The model under review builds one solid part; all positions refer to its coordinate system, in mm. Face numbers are marked on the shaded views. A direction names the side the tool comes from. Coordinates: 2 decimals unless noted, no trailing zeros. Order: outer loops, then holes, each group sorted by start corner. A loop starts at its lowest first (then second) coordinate and runs counter-clockwise, first axis right, second up. Notation, with made-up numbers: (-35.75, 38.5) - (5.25, 38.5) arc R33 cw to (5.25, 71.5) - close; hole circle Ø5 at (-33.5, 80). An arc over 180 degrees is marked (long way). Answer in a Markdown table with one row per item.
```python
from build123d import *

# Parameters (mm, degrees)
SKETCH1_W                = 47.8
SKETCH1_H                = 47.8
SKETCH1_W_2              = 40.2
SKETCH1_H_2              = 40.2
BOSS_EXTRUDE1_DEPTH      = 11
SKETCH3_W                = 20
SKETCH3_H                = 6
CUT_EXTRUDE1_DEPTH       = 55.562349656
SKETCH4_W                = 5
SKETCH4_H                = 6
CUT_EXTRUDE2_DEPTH       = 1
CUT_EXTRUDE4_REACH       = 56.562
SKETCH6_R                = 1.35
CUT_EXTRUDE5_REACH       = 56.562
SKETCH7_R                = 1.35
CUT_EXTRUDE6_REACH       = 56.562
SKETCH8_R                = 1.35
CUT_EXTRUDE7_REACH       = 56.562
SKETCH9_R                = 1.65
BOSS_EXTRUDE7_DEPTH      = 8
BOSS_EXTRUDE7_DEPTH_BACK = 10
SKETCH5_W                = 5
SKETCH5_H                = 6
CUT_EXTRUDE3_DEPTH       = 1.2
SKETCH11_R               = 2.6
CUT_EXTRUDE8_DEPTH       = 2


with BuildPart() as part:
    # Sketch1 → Boss-Extrude1 (new body)
    with BuildSketch(Plane(origin=(0, 0, 0), x_dir=(1, 0, 0), z_dir=(0, 1, 0))):
        Rectangle(SKETCH1_W, SKETCH1_H)
        Rectangle(SKETCH1_W_2, SKETCH1_H_2, mode=Mode.SUBTRACT)
    extrude(amount=BOSS_EXTRUDE1_DEPTH)

    # Sketch3 → Cut-Extrude1 (cut, through all)
    with BuildSketch(Plane.XY.offset(23.9)):
        with Locations((0, 3)):
            Rectangle(SKETCH3_W, SKETCH3_H)
    extrude(amount=-CUT_EXTRUDE1_DEPTH, mode=Mode.SUBTRACT)

    # Sketch4 → Cut-Extrude2 (cut)
    with BuildSketch(Plane.XY.offset(-20.1)):
        with Locations((-12.5, 3)):
            Rectangle(SKETCH4_W, SKETCH4_H)
        with Locations((12.5, 3)):
            Rectangle(SKETCH4_W, SKETCH4_H)
    extrude(amount=-CUT_EXTRUDE2_DEPTH, mode=Mode.SUBTRACT)

    # Sketch6 → Cut-Extrude4 (cut, up to next)
    with BuildSketch(Plane(origin=(0, 0, -23.9), x_dir=(-1, 0, 0), z_dir=(0, 0, -1)), mode=Mode.PRIVATE) as cut_extrude4_sk1:
        with Locations((-8.9, 9)):
            Circle(SKETCH6_R)
    cut_extrude4_tool1 = extrude(cut_extrude4_sk1.sketch, amount=-CUT_EXTRUDE4_REACH, mode=Mode.PRIVATE) & part.part
    # Sketch6 → Cut-Extrude4 (cut, up to next)
    with BuildSketch(Plane(origin=(0, 0, -23.9), x_dir=(-1, 0, 0), z_dir=(0, 0, -1)), mode=Mode.PRIVATE) as cut_extrude4_sk2:
        with Locations((8.9, 9)):
            Circle(SKETCH6_R)
    cut_extrude4_tool2 = extrude(cut_extrude4_sk2.sketch, amount=-CUT_EXTRUDE4_REACH, mode=Mode.PRIVATE) & part.part
    add(cut_extrude4_tool1.solids().sort_by_distance((8.9, 9, -23.9))[0], mode=Mode.SUBTRACT)
    add(cut_extrude4_tool2.solids().sort_by_distance((-8.9, 9, -23.9))[0], mode=Mode.SUBTRACT)

    # Sketch7 → Cut-Extrude5 (cut, up to next)
    with BuildSketch(Plane.XY.offset(23.9), mode=Mode.PRIVATE) as cut_extrude5_sk1:
        with Locations((9.4, 8.412816521)):
            Circle(SKETCH7_R)
    cut_extrude5_tool1 = extrude(cut_extrude5_sk1.sketch, amount=-CUT_EXTRUDE5_REACH, mode=Mode.PRIVATE) & part.part
    # Sketch7 → Cut-Extrude5 (cut, up to next)
    with BuildSketch(Plane.XY.offset(23.9), mode=Mode.PRIVATE) as cut_extrude5_sk2:
        with Locations((-5.6, 8.412816521)):
            Circle(SKETCH7_R)
    cut_extrude5_tool2 = extrude(cut_extrude5_sk2.sketch, amount=-CUT_EXTRUDE5_REACH, mode=Mode.PRIVATE) & part.part
    add(cut_extrude5_tool1.solids().sort_by_distance((9.4, 8.412817, 23.9))[0], mode=Mode.SUBTRACT)
    add(cut_extrude5_tool2.solids().sort_by_distance((-5.6, 8.412817, 23.9))[0], mode=Mode.SUBTRACT)

    # Sketch8 → Cut-Extrude6 (cut, up to next)
    with BuildSketch(Plane(origin=(23.9, 0, 0), x_dir=(0, 0, -1), z_dir=(1, 0, 0)), mode=Mode.PRIVATE) as cut_extrude6_sk1:
        with Locations((-11.9, 4)):
            Circle(SKETCH8_R)
    cut_extrude6_tool1 = extrude(cut_extrude6_sk1.sketch, amount=-CUT_EXTRUDE6_REACH, mode=Mode.PRIVATE) & part.part
    # Sketch8 → Cut-Extrude6 (cut, up to next)
    with BuildSketch(Plane(origin=(23.9, 0, 0), x_dir=(0, 0, -1), z_dir=(1, 0, 0)), mode=Mode.PRIVATE) as cut_extrude6_sk2:
        with Locations((-6.4, 4)):
            Circle(SKETCH8_R)
    cut_extrude6_tool2 = extrude(cut_extrude6_sk2.sketch, amount=-CUT_EXTRUDE6_REACH, mode=Mode.PRIVATE) & part.part
    # Sketch8 → Cut-Extrude6 (cut, up to next)
    with BuildSketch(Plane(origin=(23.9, 0, 0), x_dir=(0, 0, -1), z_dir=(1, 0, 0)), mode=Mode.PRIVATE) as cut_extrude6_sk3:
        with Locations(Location((6.4, 4, 0), (0, 0, 180))):
            Circle(SKETCH8_R)
    cut_extrude6_tool3 = extrude(cut_extrude6_sk3.sketch, amount=-CUT_EXTRUDE6_REACH, mode=Mode.PRIVATE) & part.part
    # Sketch8 → Cut-Extrude6 (cut, up to next)
    with BuildSketch(Plane(origin=(23.9, 0, 0), x_dir=(0, 0, -1), z_dir=(1, 0, 0)), mode=Mode.PRIVATE) as cut_extrude6_sk4:
        with Locations(Location((11.9, 4, 0), (0, 0, 180))):
            Circle(SKETCH8_R)
    cut_extrude6_tool4 = extrude(cut_extrude6_sk4.sketch, amount=-CUT_EXTRUDE6_REACH, mode=Mode.PRIVATE) & part.part
    add(cut_extrude6_tool1.solids().sort_by_distance((23.9, 4, 11.9))[0], mode=Mode.SUBTRACT)
    add(cut_extrude6_tool2.solids().sort_by_distance((23.9, 4, 6.4))[0], mode=Mode.SUBTRACT)
    add(cut_extrude6_tool3.solids().sort_by_distance((23.9, 4, -6.4))[0], mode=Mode.SUBTRACT)
    add(cut_extrude6_tool4.solids().sort_by_distance((23.9, 4, -11.9))[0], mode=Mode.SUBTRACT)

    # Sketch9 → Cut-Extrude7 (cut, up to next)
    with BuildSketch(Plane.ZY.offset(23.9), mode=Mode.PRIVATE) as cut_extrude7_sk1:
        with Locations((0, 6)):
            Circle(SKETCH9_R)
    cut_extrude7_tool1 = extrude(cut_extrude7_sk1.sketch, amount=-CUT_EXTRUDE7_REACH, mode=Mode.PRIVATE) & part.part
    add(cut_extrude7_tool1.solids().sort_by_distance((-23.9, 6, 0))[0], mode=Mode.SUBTRACT)

    # Sketch10 → Boss-Extrude7 (add, two sides: drawn at the far end of the back side and taken through both)
    with BuildSketch(Plane(origin=(23.9, 0, 0), x_dir=(0, 0, -1), z_dir=(1, 0, 0)).offset(-BOSS_EXTRUDE7_DEPTH_BACK)):
        with BuildLine():
            Line((-42.1, 0), (-20.1, 0))
            Line((-20.1, 0), (-20.1, 11))
            Line((-20.1, 11), (-25.535668372, 21.478172171))
            ThreePointArc((-25.535668372, 21.478172171), (-32.693052351, 5.7261976), (-46.3, 16.412816521))
            Line((-46.3, 16.412816521), (-46.3, 8.096211929))
            Line((-46.3, 8.096211929), (-42.1, 0))
        make_face()
        with BuildLine():
            ThreePointArc((-46.3, 16.412816521), (-32.693052351, 5.7261976), (-25.535668372, 21.478172171))
            Line((-25.535668372, 21.478172171), (-26.423334884, 21.017685293))
            ThreePointArc((-26.423334884, 21.017685293), (-32.930047592, 6.697708411), (-45.3, 16.412816521))
            Line((-45.3, 16.412816521), (-46.3, 16.412816521))
        make_face()
    extrude(amount=BOSS_EXTRUDE7_DEPTH + BOSS_EXTRUDE7_DEPTH_BACK)

    # Sketch5 → Cut-Extrude3 (cut)
    with BuildSketch(Plane(origin=(0, 0, 20.1), x_dir=(-1, 0, 0), z_dir=(0, 0, -1))):
        with Locations((-12.5, 3)):
            Rectangle(SKETCH5_W, SKETCH5_H)
        with Locations((12.5, 3)):
            Rectangle(SKETCH5_W, SKETCH5_H)
    extrude(amount=-CUT_EXTRUDE3_DEPTH, mode=Mode.SUBTRACT)

    # Sketch11 → Cut-Extrude8 (cut)
    with BuildSketch(Plane(origin=(23.9, 0, 0), x_dir=(0, 0, -1), z_dir=(1, 0, 0))):
        with Locations((11.9, 4)):
            Circle(SKETCH11_R)
        with Locations((6.4, 4)):
            Circle(SKETCH11_R)
        with Locations((-6.4, 4)):
            Circle(SKETCH11_R)
        with Locations((-11.9, 4)):
            Circle(SKETCH11_R)
    extrude(amount=-CUT_EXTRUDE8_DEPTH, mode=Mode.SUBTRACT)


solid = part.part
```
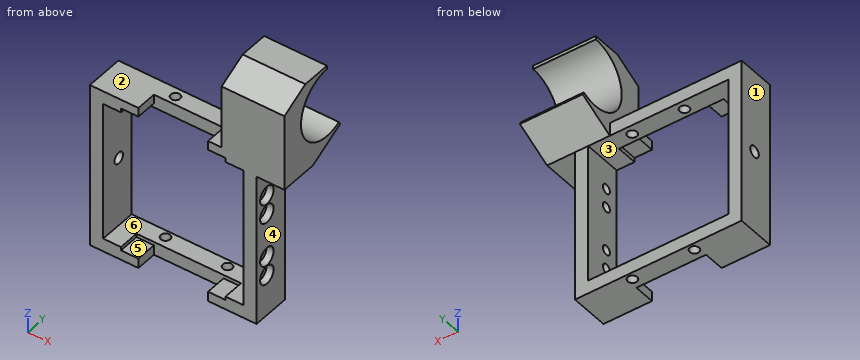
Item 1: We need section C-C, the plane z = 11.9. Write out the cut boundary in (x, y).
Check values:
| item | result |
|---|---|
| outline | (-23.9, 0) - (-20.1, 0) - (-20.1, 11) - (-23.9, 11) - close; (20.1, 0) - (23.9, 0) - (23.9, 1.4) - (21.9, 1.4) - (21.9, 2.65) - (20.1, 2.65) - close; (20.1, 5.35) - (21.9, 5.35) - (21.9, 6.6) - (23.9, 6.6) - (23.9, 11) - (20.1, 11) - close |
Item 2: Clearance check with flat-ended pins moving along their axes: pin 1 Ø10 at (y, z) = (8, 30.5) entering from -X; pin 2 Ø9 at (x, y) = (0, 8) entering from +Z; pin 3 Ø12 at (y, z) = (16, -15.5) entering from +X. State where each tip first meets the part, or that it passes through.
Check values:
| item | result |
|---|---|
| pin 1 | x = 13.9 |
| pin 2 | z = 23.9 |
| pin 3 | x = 23.9 |
Item 3: We need section A-A, the plane z = -15.5. Write out the cut boundary in (x, y).
Check values:
| item | result |
|---|---|
| outline | (-23.9, 0) - (-20.1, 0) - (-20.1, 11) - (-23.9, 11) - close; (20.1, 0) - (23.9, 0) - (23.9, 11) - (20.1, 11) - close |
Item 4: Mouldability with a two-part tool opening along X and no side actions: class the marked faces 1, 2 and 3 as +X half, -X half, draft (parallel to the pull), parting line (faces both ways), or undercut.
Check values:
| item | result |
|---|---|
| face 1 | -X half |
| face 2 | draft |
| face 3 | undercut |
Item 5: Tool access review of the marked faces 4, 5 and 6: name each direction out of +Z, -Z, +X, -X, +Y, -Y from which nothing blocks a thin tool from reaching the whole face with its end or side.
Check values:
| item | result |
|---|---|
| face 4 | -Z, +X, +Y, -Y |
| face 5 | -Y |
| face 6 | +Y, -Y |
Item 6: We need section D-D, the plane x = -5.5. Write out the cut boundary in (y, z).
Check values:
| item | result |
|---|---|
| outline | (6, -23.9) - (11, -23.9) - (11, -20.1) - (6, -20.1) - close; (6, 20.1) - (7.07, 20.1) - (7.07, 23.9) - (6, 23.9) - close; (9.76, 20.1) - (11, 20.1) - (11, 23.9) - (9.76, 23.9) - close |
Item 7: We need section B-B, the plane x = 5.5. Write out the cut boundary in (y, z).
Check values:
| item | result |
|---|---|
| outline | (6, -23.9) - (11, -23.9) - (11, -20.1) - (6, -20.1) - close; (6, 20.1) - (11, 20.1) - (11, 23.9) - (6, 23.9) - close |
Item 8: To check wall thickness, follow line 1 (Y direction, x = 8.9, z = -21.6); line 2 (Z direction, x = 11, y = 8.75). State the ranges of each line that lie inside material, in increasing order. Write a range as from..to.
Check values:
| item | result |
|---|---|
| line 1 | 6..7.65, 10.35..11 |
| line 2 | -23.9..-20.1, 20.1..23.9 |
